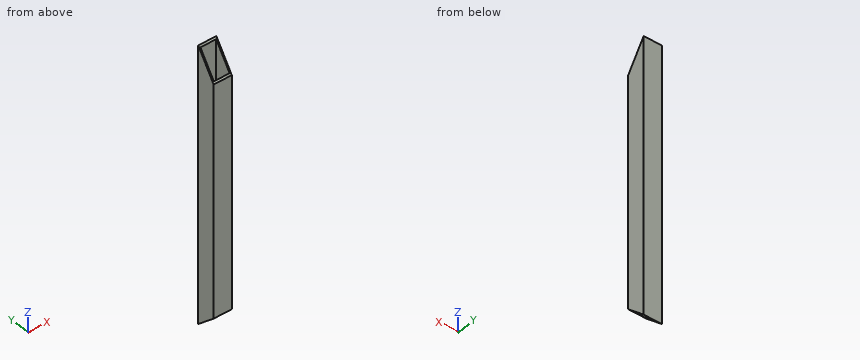
from build123d import *

# Parameters (mm, degrees)
SKETCH1_W           = 25.4
SKETCH1_H           = 25.4
SKETCH1_W_2         = 22.098
SKETCH1_H_2         = 22.098
BOSS_EXTRUDE1_DEPTH = 378.309163
CUT_EXTRUDE2_DEPTH  = 26.4
SKETCH5_W           = 25.4
SKETCH5_H           = 25.4
CUT_EXTRUDE3_DEPTH  = 244.121498097


with BuildPart() as part:
    # Sketch1 → Boss-Extrude1 (new body)
    with BuildSketch(Plane.XY):
        Rectangle(SKETCH1_W, SKETCH1_H)
        Rectangle(SKETCH1_W_2, SKETCH1_H_2, mode=Mode.SUBTRACT)
    extrude(amount=BOSS_EXTRUDE1_DEPTH)

    # Sketch4 → Cut-Extrude2 (cut, through all)
    with BuildSketch(Plane.ZY.offset(12.7)):
        Polygon((0, 12.7), (22.23162961, -12.749147595), (0, -16.391086304), align=None)
    extrude(amount=-CUT_EXTRUDE2_DEPTH, mode=Mode.SUBTRACT)

    # Sketch5 → Cut-Extrude3 (cut, through all)
    with BuildSketch(Plane(origin=(0, -132.21706056, 182.766862758), x_dir=(1, 0, 0), z_dir=(0, 0.557172611, 0.830396701))):
        Rectangle(SKETCH5_W, SKETCH5_H)
    extrude(amount=CUT_EXTRUDE3_DEPTH, mode=Mode.SUBTRACT)


solid = part.part
Read the model definition and answer for the solid it produces. Units are mm, in the model's axes. Round coordinates to 2 decimals unless told otherwise and drop trailing zeros. Write each loop counter-clockwise with the first axis right and the second up, starting at its lowest first coordinate (ties: lowest second). Pieces come first, ordered by that corner, then holes. Notation, with made-up numbers: (36, -14.5) - (61, -14.5) arc R14 ccw to (61, 9.5) - close; hole circle Ø5 at (-27.5, -23.75). An arc over 180 degrees is marked (long way). One line per question, with ' | ' between items. Start each with the question number.
1. Section C-C (y = -5) is taken. Determine the outline of the cut face in (x, z).
2. Section B-B (z = 244) is taken. Determine the outline of the cut face in (x, y).
3. Section A-A (x = 3.5) is taken. Determine the outline of the cut face in (y, z).
4. Find the intervals of material crossed by probe 1 along X at (y, z) = (-9.75, 258.5); probe 2 along Y at (x, z) = (10.5, 347), in increasing order. Write a range as [from, to].
Filled in:
1) outline: (-12.7, 15.46) - (-11.05, 15.46) - (-11.05, 349.57) - (-12.7, 349.57) - close; (11.05, 15.46) - (12.7, 15.46) - (12.7, 349.57) - (11.05, 349.57) - close
2) outline: (-12.7, -12.7) - (12.7, -12.7) - (12.7, 12.7) - (-12.7, 12.7) - close; hole (-11.05, -11.05) - (11.05, -11.05) - (11.05, 11.05) - (-11.05, 11.05) - close
3) outline: (-12.7, 22.19) - (-11.05, 20.75) - (-11.05, 340.56) - (-12.7, 338.1) - close; (11.05, 1.44) - (12.7, 0) - (12.7, 375.95) - (11.05, 373.49) - close
4) probe 1: [-12.7, -11.05], [11.05, 12.7] | probe 2: [11.05, 12.7]
